Autodesk Fusion 360 part; units mm, degrees
sketch "Sketch1" plane through (0, 0, 0) normal (0, 0, 1) x (1, 0, 0)
  circle A0 centre (0, 0) radius 10
  circle A1 centre (0, 0) radius 14
  dimension "d1" = 20
  dimension "d2" = 28
extrude "Extrude3" add sketch "Sketch1" along normal blind 7 contours A0 | A1 makes body 1
extrude "Extrude2" add sketch "Sketch1" along normal blind 8 separate body contours A0 makes body 2
extrude "Extrude1" add sketch "Sketch1" along normal blind 40 separate body makes body 3
fillet "Fillet1" radius 3 1 edges at (-13.0526, -5.0626, 40) on bodies 3
combine "Combine1" operation add target body 3 tool bodies 1 2
sketch "Sketch2" plane through (0, 0, 0) normal (0, 1, 0) x (1, 0, 0)
  circle A0 centre (0, -26) radius 1.4
  circle A1 centre (0, -26) radius 4.4
  dimension "d10" = 2.8
  dimension "d11" = 3
extrude "Extrude5" cut sketch "Sketch2" along normal up to surface contours A0 end surface at (13.9304, -1.3939, 12.3333) on bodies 3 bodies 3
extrude "Extrude4" add sketch "Sketch2" along normal up to surface and the other way blind -16 end surface at (-2.9183, -9.5647, 24.6793) on bodies 3 bodies 3
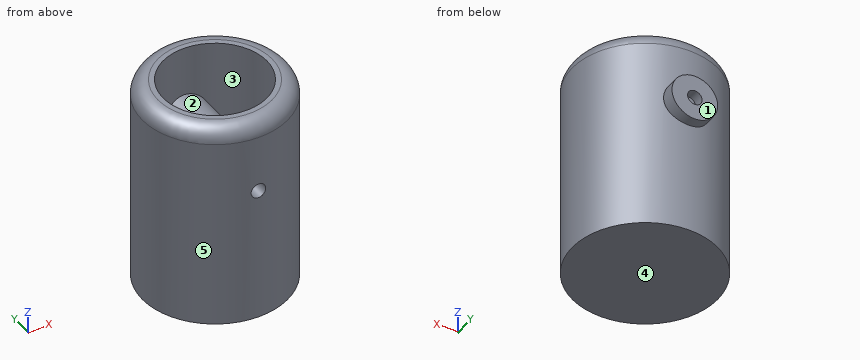
Design review of the part built by this model. Coordinates are the model's own, in mm. Face numbers are marked on the shaded views. A direction names the side the tool comes from. Give positions to 0.01 mm unless a question says otherwise; leave off trailing zeros. Write each loop counter-clockwise with the first axis right and the second up, starting at its lowest first coordinate (ties: lowest second). Pieces come first, ordered by that corner, then holes. Notation, with made-up numbers: (0, -28.5) - (45, -28.5) arc R29 cw to (45, 7.5) - close; hole circle Ø6 at (68.5, 61.25). An arc over 180 degrees is marked (long way). Return JSON: item names as keys, results as strings. Group by question number.
(1) We need section C-C, the plane z = 19.5. Give the boundary of the cut face in (x, y), then the cut area to 3 significant figures.
(2) We need section B-B, the plane x = 0. Give the boundary of the cut face in (y, z), then the cut area to 3 significant figures.
(3) We need section D-D, the plane z = 26. Give the boundary of the cut face in (x, y), then the cut area to 3 significant figures.
(4) Insertion check: pin 1 (6 mm diameter, centred on y = -2, z = 33, fed in from -X); pin 2 (8 mm diameter, centred on y = 7.5, z = 7.5, fed in from -X); pin 3 (1 mm diameter, centred on y = 2, z = 31.5, fed in from -X); pin 4 (1.5 mm diameter, centred on x = 9.5, z = 16.5, fed in from +Y). Each pin has a flat end and moves straight along its axis. Give the tip position at first contact, or say it passes through.
(5) Machinability: for the marked faces 1 and 2, which of the approach directions +Z, -Z, +X, -X, +Y, -Y give a long, thin tool a straight path to every point of the face, cutting with its end or side? Answer none if there is none.
(6) To check wall thickness, follow probe 1 along Z at (x, y) = (0, -1.75); probe 2 along X at (y, z) = (14.6, 26); probe 3 along X at (y, z) = (-5, 23). State the ranges of each line that lie inside material, in increasing order.
(7) We need section A-A, the plane y = 0. Give the boundary of the cut face in (x, z), then the cut area to 3 significant figures.
(8) Mouldability with a two-part tool opening along X and no side actions: class the marked faces 3, 4 and 5 as +X half, -X half, draft (parallel to the pull), parting line (faces both ways), or undercut.
Reported:
{
 "1": {"outline": "circle Ø28 at (0, 0); hole circle Ø20 at (0, 0)", "area": "302 mm2"},
 "2": {"outline": "(-14, 0) - (14, 0) - (14, 21.6) - (16, 21.6) - (16, 24.6) - (14, 24.6) - (14, 27.4) - (16, 27.4) - (16, 30.4) - (14, 30.4) - (14, 37) arc R3 ccw to (11, 40) - (10, 40) - (10, 30.4) - (-10, 30.4) - (-10, 40) - (-11, 40) arc R3 ccw to (-14, 37) - (-14, 27.4) - (10, 27.4) - (10, 24.6) - (-14, 24.6) - close; hole (-10, 8) - (10, 8) - (10, 21.6) - (-10, 21.6) - close", "area": "597 mm2"},
 "3": {"outline": "(-4.4, 13.29) arc R14 ccw to (-1.4, -13.93) - (-1.4, 9.9) arc R10 cw to (1.4, 9.9) - (1.4, -13.93) arc R14 ccw to (4.4, 13.29) - (4.4, 16) - (1.4, 16) - (1.4, 13.93) arc R14 ccw to (-1.4, 13.93) - (-1.4, 16) - (-4.4, 16) - close; hole (-4.4, -8.98) - (-4.4, 8.98) arc R10 ccw to start; hole (4.4, -8.98) arc R10 ccw to (4.4, 8.98) - close", "area": "419 mm2"},
 "4": {"pin 1": "stops at x = -14", "pin 2": "stops at x = -13.56", "pin 3": "stops at x = -13.92", "pin 4": "stops at y = 10.93"},
 "5": {"face 1": "+Z, -Z, +X, -X, +Y", "face 2": "none"},
 "6": {"probe 1": "z = 0 to 8, 21.6 to 24.6, 27.4 to 30.4", "probe 2": "x = -4.4 to -1.4, 1.4 to 4.4", "probe 3": "x = -13.08 to -8.66, -3.22 to 3.22, 8.66 to 13.08"},
 "7": {"outline": "(-14, 0) - (14, 0) - (14, 37) arc R3 ccw to (11, 40) - (10, 40) - (10, 8) - (-10, 8) - (-10, 40) - (-11, 40) arc R3 ccw to (-14, 37) - close; circle Ø8.8 at (0, 26); hole circle Ø2.8 at (0, 26)", "area": "531 mm2"},
 "8": {"face 3": "undercut", "face 4": "draft", "face 5": "parting line"}
}
